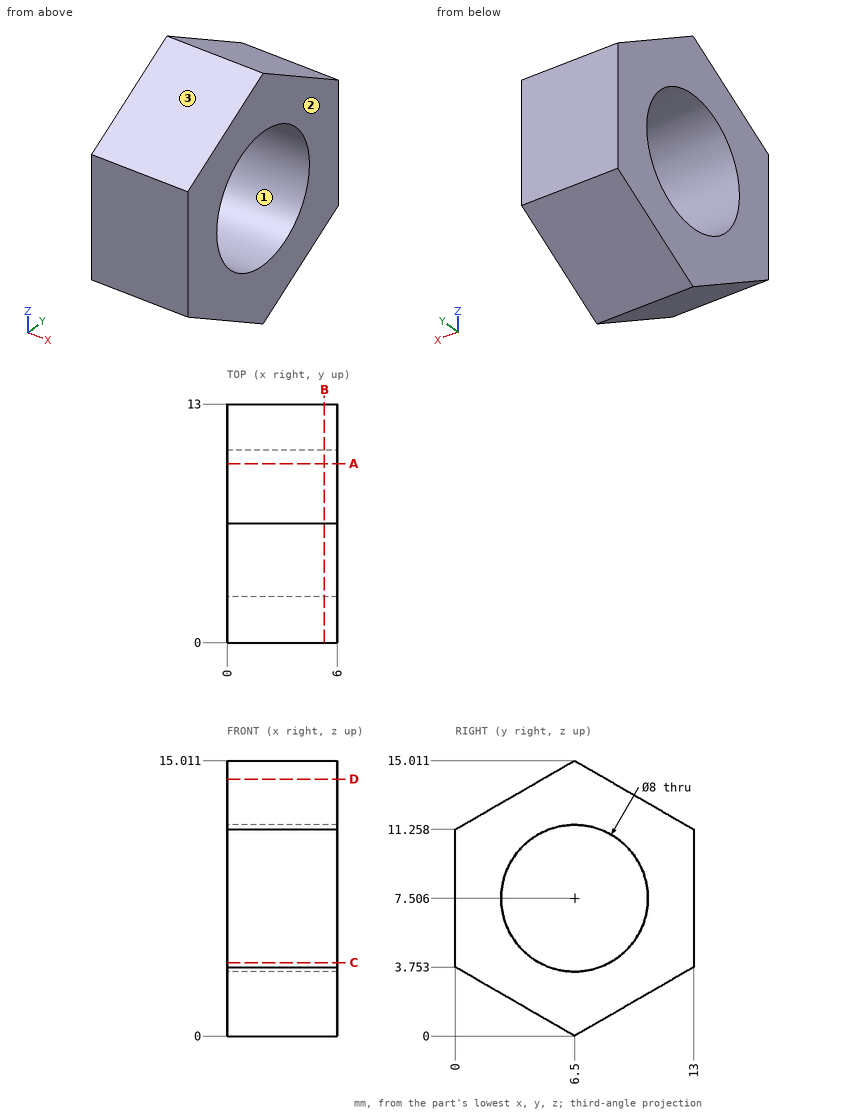
Source: three-view drawing plus pictorial views. Frame: mm from the lowest corner of the part. Round coordinates to 2 decimals unless told otherwise and drop trailing zeros. Loops run counter-clockwise (first coordinate to the right, second up) from the corner with the lowest first, then second, coordinate; pieces in that order, holes last. Notation, with made-up numbers: M -24,52 L 16,52 A7 ccw 16,60 Z; hole C 69.5,62.5 d2. An arc over 180 degrees is marked long. Answer as CSV lines item,"result". Start each with the question number.
(1) Section D-D, the plane z = 14. Output: boundary loops of the cut face in (x, y), plus the area to 3 significant figures.
(2) Section C-C, the plane z = 4. Output: boundary loops of the cut face in (x, y).
(3) Draft query along Y for the marked faces 1, 2 and 3. Return one class per face: released by +Y, released by -Y, zero draft, split by the parting line, or undercut.
(4) Line query: line 1 (Y direction, x = 3.2, z = 5.5); line 2 (Z direction, x = 5.7, y = 5.25) (1 decimal); line 3 (Y direction, x = 3.45, z = 10.5). Output: solid intervals per line, ascending. Write a range as [from, to].
(5) First-contact query: pin 1 (3 mm diameter, centred on x = 4, y = 2.5, fed in from -Z); pin 2 (7 mm diameter, centred on y = 6.5, z = 7.51, fed in from -X). Flat tips, straight axial feed; report the tip coordinate or a pass-through.
(6) Section A-A, the plane y = 9.75. Output: boundary loops of the cut face in (x, z) (1 decimal).
(7) Section B-B, the plane x = 5.3. Output: boundary loops of the cut face in (y, z) (1 decimal).
Values found:
1,outline,"M 0,4.75 L 6,4.75 L 6,8.25 L 0,8.25 Z"
1,area,"21.0 mm²"
2,outline,"M 0,0 L 6,0 L 6,4.57 L 0,4.57 Z; M 0,8.43 L 6,8.43 L 6,13 L 0,13 Z"
3,face 1,"undercut"
3,face 2,"zero draft"
3,face 3,"released by -Y"
4,line 1,"y = [0, 3.04], [9.96, 13]"
4,line 2,"z = [0.7, 3.7], [11.3, 14.3]"
4,line 3,"y = [0, 3.85], [9.15, 13]"
5,pin 1,"stops at z = 1.44"
5,pin 2,"passes through"
6,outline,"M 0,1.9 L 6,1.9 L 6,5.2 L 0,5.2 Z; M 0,9.8 L 6,9.8 L 6,13.1 L 0,13.1 Z"
7,outline,"M 0,3.8 L 6.5,0 L 13,3.8 L 13,11.3 L 6.5,15 L 0,11.3 Z; hole C 6.5,7.5 d8"
